Build history of the part. All positions in model axes, mm. Round coordinates to 2 decimals unless told otherwise and drop trailing zeros. Write each loop counter-clockwise with the first axis right and the second up, starting at its lowest first coordinate (ties: lowest second). Pieces come first, ordered by that corner, then holes.
1) Saw through at B-B (z = 2.25). Write the cut outline in (x, y), plus the area to 3 significant figures.
2) Wall check: probe 1 along Y at (x, z) = (3, 2.65); probe 2 along Z at (x, y) = (2, 2); probe 3 along Z at (x, y) = (5.5, 1.25). Give the ranges that are in metal, low to high.
3) Saw through at C-C (y = 1). Write the cut outline in (x, z).
from build123d import *

# Parameters (mm, degrees)
SKETCH1_W           = 8
SKETCH1_H           = 7
BOSS_EXTRUDE1_DEPTH = 4
FILLET1_R           = 3.5


with BuildPart() as part:
    # Sketch1 → Boss-Extrude1 (new body)
    with BuildSketch(Plane.XY):
        with Locations((4, 3.5)):
            Rectangle(SKETCH1_W, SKETCH1_H)
    extrude(amount=BOSS_EXTRUDE1_DEPTH)

    # Fillet1
    fillet1_edges = [part.edges().sort_by_distance(p)[0] for p in [
        (4, 0, 4),
        (4, 7, 4),
    ]]
    fillet(fillet1_edges, radius=FILLET1_R - 0.0001)  # a hair under: the kernel refuses the full size


solid = part.part
Evaluation:
1. outline: (0, 0.47) - (8, 0.47) - (8, 6.53) - (0, 6.53) - close
1. area: 48.5 mm2
2. probe 1: y = 0.74 to 6.26
2. probe 2: z = 0 to 3.66
2. probe 3: z = 0 to 3.18
3. outline: (0, 0) - (8, 0) - (8, 2.95) - (0, 2.95) - close
